```python
from build123d import *

# Parameters (mm, degrees)
SKETCH1_W                      = 160
SKETCH1_H                      = 32
BOSS_EXTRUDE1_DEPTH            = 32
SKETCH2_W                      = 28
SKETCH2_H                      = 30
CUT_EXTRUDE1_DEPTH             = 161
F_8_0_8_DIAMETER_HOLE1_D       = 8
F_8_0_8_DIAMETER_HOLE1_DEPTH   = 2
F_3_7_3_7_DIAMETER_HOLE1_D     = 3.7
F_3_7_3_7_DIAMETER_HOLE1_DEPTH = 2
F_3_7_3_7_DIAMETER_HOLE2_D     = 3.7
F_3_7_3_7_DIAMETER_HOLE2_DEPTH = 32
F_8_0_8_DIAMETER_HOLE2_D       = 8
F_8_0_8_DIAMETER_HOLE2_DEPTH   = 32
F_8_0_8_DIAMETER_HOLE3_D       = 8
F_8_0_8_DIAMETER_HOLE3_DEPTH   = 2
F_8_0_8_DIAMETER_HOLE4_D       = 8
F_8_0_8_DIAMETER_HOLE4_DEPTH   = 32
F_3_7_3_7_DIAMETER_HOLE3_D     = 3.7
F_3_7_3_7_DIAMETER_HOLE3_DEPTH = 32
FILLET1_R                      = 2.5


with BuildPart() as part:
    # Sketch1 → Boss-Extrude1 (new body)
    with BuildSketch(Plane(origin=(16, 0, 0), x_dir=(0, 0, -1), z_dir=(1, 0, 0))):
        with Locations((64, 16)):
            Rectangle(SKETCH1_W, SKETCH1_H)
    extrude(amount=-BOSS_EXTRUDE1_DEPTH)

    # Sketch2 → Cut-Extrude1 (cut, through all)
    with BuildSketch(Plane(origin=(0, 0, -144), x_dir=(-1, 0, 0), z_dir=(0, 0, -1))):
        with Locations((0, 17)):
            Rectangle(SKETCH2_W, SKETCH2_H)
    extrude(amount=-CUT_EXTRUDE1_DEPTH, mode=Mode.SUBTRACT)

    # Ø8.0 (8) Diameter Hole1
    with Locations(Plane.ZY.offset(16)):
        with Locations((-64, 16), (-128, 16), (-32, 16), (-96, 16), (-16, 16), (-48, 16), (-80, 16), (-112, 16), (0, 16)):
            Hole(F_8_0_8_DIAMETER_HOLE1_D / 2, depth=F_8_0_8_DIAMETER_HOLE1_DEPTH)

    # Ø3.7 (3.7) Diameter Hole1
    with Locations(Plane.ZY.offset(16)):
        with Locations((0, 24), (0, 8), (-8, 16), (8, 16), (-5.656854249, 21.656854249), (5.656854249, 21.656854249), (5.656854249, 10.343145751), (-5.656854249, 10.343145751), (-64, 24), (-64, 8), (-72, 16), (-56, 16), (-69.656854249, 21.656854249), (-58.343145751, 21.656854249), (-58.343145751, 10.343145751), (-69.656854249, 10.343145751), (-128, 24), (-128, 8), (-136, 16), (-120, 16), (-133.656854249, 21.656854249), (-122.34314575, 21.656854249), (-122.34314575, 10.343145751), (-133.656854249, 10.343145751), (-32, 24), (-40, 16), (-32, 8), (-24, 16), (-96, 24), (-104, 16), (-96, 8), (-88, 16)):
            Hole(F_3_7_3_7_DIAMETER_HOLE1_D / 2, depth=F_3_7_3_7_DIAMETER_HOLE1_DEPTH)

    # Ø3.7 (3.7) Diameter Hole2
    with Locations(Plane(origin=(0, 0, 0), x_dir=(-1, 0, 0), z_dir=(0, -1, 0))):
        with Locations((8, 0), (5.656854249, 5.656854249), (0, 8), (-5.656854249, 5.656854249), (-8, 0), (-5.656854249, -5.656854249), (0, -8), (5.656854249, -5.656854249), (8, 64), (5.656854249, 69.656854249), (0, 72), (-5.656854249, 69.656854249), (-8, 64), (-5.656854249, 58.343145751), (0, 56), (5.656854249, 58.343145751), (8, 128), (5.656854249, 133.656854249), (0, 136), (-5.656854249, 133.656854249), (-8, 128), (-5.656854249, 122.34314575), (0, 120), (5.656854249, 122.34314575), (8, 32), (0, 40), (-8, 32), (0, 24), (8, 96), (0, 104), (-8, 96), (0, 88)):
            Hole(F_3_7_3_7_DIAMETER_HOLE2_D / 2, depth=F_3_7_3_7_DIAMETER_HOLE2_DEPTH)

    # Ø8.0 (8) Diameter Hole2
    with Locations(Plane(origin=(0, 0, 0), x_dir=(-1, 0, 0), z_dir=(0, -1, 0))):
        with Locations((0, 0), (0, 64), (0, 128), (0, 32), (0, 96), (0, 16), (0, 48), (0, 80), (0, 112)):
            Hole(F_8_0_8_DIAMETER_HOLE2_D / 2, depth=F_8_0_8_DIAMETER_HOLE2_DEPTH)

    # Ø8.0 (8) Diameter Hole3
    with Locations(Plane.ZY.offset(-14)):
        with Locations((-32, 16)):
            Hole(F_8_0_8_DIAMETER_HOLE3_D / 2, depth=F_8_0_8_DIAMETER_HOLE3_DEPTH)

    # Ø8.0 (8) Diameter Hole4
    with Locations(Plane(origin=(16, 0, 0), x_dir=(0, 0, -1), z_dir=(1, 0, 0))):
        with Locations((64, 16), (128, 16), (96, 16), (16, 16), (48, 16), (80, 16), (112, 16), (0, 16)):
            Hole(F_8_0_8_DIAMETER_HOLE4_D / 2, depth=F_8_0_8_DIAMETER_HOLE4_DEPTH)

    # Ø3.7 (3.7) Diameter Hole3
    with Locations(Plane(origin=(16, 0, 0), x_dir=(0, 0, -1), z_dir=(1, 0, 0))):
        with Locations((0, 24), (0, 8), (8, 16), (-8, 16), (5.656854249, 21.656854249), (-5.656854249, 21.656854249), (-5.656854249, 10.343145751), (5.656854249, 10.343145751), (64, 24), (64, 8), (72, 16), (56, 16), (69.656854249, 21.656854249), (58.343145751, 21.656854249), (58.343145751, 10.343145751), (69.656854249, 10.343145751), (128, 24), (128, 8), (136, 16), (120, 16), (133.656854249, 21.656854249), (122.34314575, 21.656854249), (122.34314575, 10.343145751), (133.656854249, 10.343145751), (32, 24), (40, 16), (32, 8), (24, 16), (96, 24), (104, 16), (96, 8), (88, 16)):
            Hole(F_3_7_3_7_DIAMETER_HOLE3_D / 2, depth=F_3_7_3_7_DIAMETER_HOLE3_DEPTH)

    # Fillet1
    fillet1_edges = [part.edges().sort_by_distance(p)[0] for p in [
        (-16, 0, -64),
        (15, 32, 16),
        (15, 32, -144),
        (16, 0, -64),
        (-15, 32, -144),
        (-15, 32, 16),
    ]]
    fillet(fillet1_edges, radius=FILLET1_R)


solid = part.part
```
The model under review builds one solid part; all positions refer to its coordinate system, in mm. Coordinates: 2 decimals unless noted, no trailing zeros. Write each loop counter-clockwise with the first axis right and the second up, starting at its lowest first coordinate (ties: lowest second). Pieces come first, ordered by that corner, then holes. Notation, with made-up numbers: (-6.75, -22.5) -> (52.25, -22.5) arc R17 cw to (52.25, 2.5) -> close; hole circle Ø2 at (47, -8.5). An arc over 180 degrees is marked (long way). One line per item, written item: value. Start each with the question number.
Q1. Add section A-A, the plane z = -80. Give the boundary of the cut face in (x, y), then the cut area to 3 significant figures.
Q2. Add section B-B, the plane y = 16. Count the separate pieces of the cut face and the enclosed holes in it, then the cut area to 3 significant figures.
Q3. To check wall thickness, follow probe 1 along Z at (x, y) = (-8, 1); probe 2 along X at (y, z) = (31.5, -95); probe 3 along Y at (x, z) = (15.3, 0). State the ranges of each line that lie inside material, in increasing order.
Q4. Clearance check with flat-ended pins moving along their axes: P1, Ø4.5, axis at x = 5.66, z = -122.34, coming from the +Y side; P2, Ø3.5, axis at y = 10.34, z = -5.66, coming from the -X side. State where each tip first meets the part, or that it passes through.
Response:
1. outline: (-16, 2.5) arc R2.5 ccw to (-13.5, 0) -> (-4, 0) -> (-4, 2) -> (-14, 2) -> (-14, 12) -> (-16, 12) -> close; (-16, 20) -> (-14, 20) -> (-14, 32) -> (-16, 32) -> close; (4, 0) -> (13.5, 0) arc R2.5 ccw to (16, 2.5) -> (16, 12) -> (14, 12) -> (14, 2) -> (4, 2) -> close; (14, 20) -> (16, 20) -> (16, 32) -> (14, 32) -> close
1. area: 133 mm²
2. separate pieces: 40
2. enclosed holes: 0
2. area: 204 mm²
3. probe 1: -144 to -129.85, -126.15 to -97.85, -94.15 to -65.85, -62.15 to -33.85, -30.15 to -1.85, 1.85 to 16
3. probe 2: -16 to -14, 14 to 16
3. probe 3: 0.77 to 6.15, 9.85 to 12, 20 to 22.15, 25.85 to 32
4. P1: y = 2
4. P2: through
